Can you work these out from the drawing? Everything is in mm from the part's minimum corner. A direction names the side the tool comes from. Round coordinates to 2 decimals unless told otherwise and drop trailing zeros. Loops run counter-clockwise (first coordinate to the right, second up) from the corner with the lowest first, then second, coordinate; pieces in that order, holes last. Notation, with made-up numbers: (4.5, 60) - (53.5, 60) arc R29 cw to (53.5, 97) - close; hole circle Ø7 at (-12, 58). An arc over 180 degrees is marked (long way). Answer as CSV lines item,"result". Start each with the question number.
1) Please list where these lines run through material, in increasing order: line 1 along Z through (x, y) = (1.9, 7.5); line 2 along Z through (x, y) = (2.45, 8.5); line 3 along Y through (x, z) = (2.7, 7).
2) Suppose I cut it at D-D, the plane z = 4. Write out the boundary of the cut face in (x, y), then the cut area to 3 significant figures.
3) Which directions (+Z, -Z, +X, -X, +Y, -Y) give clear straight access to the entire face, cutting with the end or side of a thin tool? Please do the marked faces 4 and 5.
4) Suppose I cut it at B-B, the plane x = 0.55. Write out the boundary of the cut face in (y, z).
5) I'm going to push flat-ended pins straight in: pin 1 Ø1.5 at (x, y) = (2, 5) entering from -Z; pin 2 Ø1.5 at (x, y) = (1, 9) entering from +Z; pin 3 Ø0.9 at (x, y) = (2, 5) entering from +Z. Where does each tip first touch, or does it pass through?
6) Suppose I cut it at A-A, the plane z = 6. Write out the boundary of the cut face in (x, y).
7) We'd pull the mould along Y, two halves only. Please class the marked faces 1, 2 and 3: pulls with the +Y half, pulls with the -Y half, needs draft (parallel to the pull), parting line crosses it, or undercut.
8) Suppose I cut it at C-C, the plane y = 7.25. Write out the boundary of the cut face in (x, z).
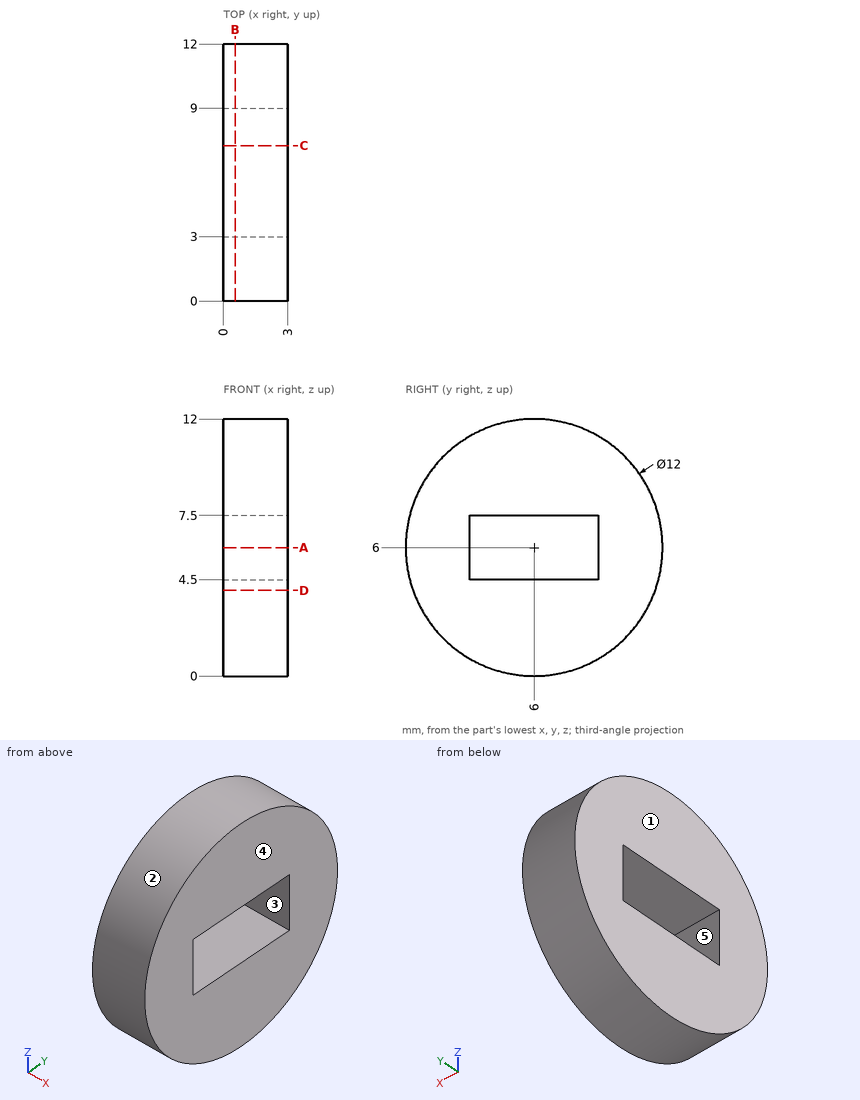
Filled sheet:
1,line 1,"0.19 to 4.5, 7.5 to 11.81"
1,line 2,"0.55 to 4.5, 7.5 to 11.45"
1,line 3,"0.08 to 3, 9 to 11.92"
2,outline,"(0, 0.34) - (3, 0.34) - (3, 11.66) - (0, 11.66) - close"
2,area,"33.9 mm²"
3,face 4,"+Z, -Z, +X, +Y, -Y"
3,face 5,"+X, -X"
4,outline,"circle Ø12 at (6, 6); hole (3, 4.5) - (9, 4.5) - (9, 7.5) - (3, 7.5) - close"
5,pin 1,"z = 0.01"
5,pin 2,"z = 11.56"
5,pin 3,"z = 11.97"
6,outline,"(0, 0) - (3, 0) - (3, 3) - (0, 3) - close; (0, 9) - (3, 9) - (3, 12) - (0, 12) - close"
7,face 1,"needs draft"
7,face 2,"parting line crosses it"
7,face 3,"undercut"
8,outline,"(0, 0.13) - (3, 0.13) - (3, 4.5) - (0, 4.5) - close; (0, 7.5) - (3, 7.5) - (3, 11.87) - (0, 11.87) - close"
